```python
from build123d import *

# Parameters (mm, degrees)
F0_W     = 25.4
F0_H     = 6.604
F1_DEPTH = 3.175
F0_H_2   = 13.716
F0_H_3   = 2.54
F2_DEPTH = 19.05
F3_R     = 12.69999
F4_R     = 1.5875
F5_DEPTH = 25.4
F6_R     = 1.5875
F7_DEPTH = 2.54


# Not quite as in the source:
# - a fillet or chamfer is up to 0.001 mm smaller than in the source, because OpenCascade refuses the exact size


with BuildPart() as f1:
    # F0 (on Top) → F1 (new body)
    with BuildSketch(Plane.XY):
        Rectangle(F0_W, F0_H)
    extrude(amount=F1_DEPTH)



with BuildPart() as f1b:
    # F0 (on Top) → F1, piece 2 (new body)
    with BuildSketch(Plane.XY):
        with Locations((0, 12.7)):
            Rectangle(F0_W, F0_H_2)
    extrude(amount=F1_DEPTH)


with BuildPart() as f1_1:
    add(f1.part)

    add(f1b.part)  # F2 merges F1b
    # F0 (on Top) → F2 (join)
    with BuildSketch(Plane.XY):
        with Locations((0, -4.572)):
            Rectangle(F0_W, F0_H_3)
        with Locations((0, 4.572)):
            Rectangle(F0_W, F0_H_3)
    extrude(amount=F2_DEPTH)

    # F3 (radius 12.7 in the source; OpenCascade refuses exactly that, so slightly less here)
    f3_edges = [f1_1.edges().sort_by_distance(p)[0] for p in [
        (12.7, -4.572, 19.05),
        (12.7, 4.572, 19.05),
        (-12.7, -4.572, 19.05),
        (-12.7, 4.572, 19.05),
        (12.7, 19.558, 1.5875),
        (-12.7, 19.558, 1.5875),
    ]]
    fillet(f3_edges, radius=F3_R)

    # F4 (on face) → F5 (cut)
    with BuildSketch(Plane.XY.offset(3.175)):
        with Locations((0, 12.7)):
            Circle(F4_R)
    extrude(amount=-F5_DEPTH, mode=Mode.SUBTRACT)

    # F6 (on face) → F7 (cut, through all)
    with BuildSketch(Plane(origin=(0, 5.842, 0), x_dir=(-1, 0, 0), z_dir=(0, 1, 0))):
        with Locations((0, 10.033)):
            Circle(F6_R)
    extrude(amount=-F7_DEPTH, mode=Mode.SUBTRACT)


solid = f1_1.part
```
The listing builds one solid part. Answer for the finished solid, in the listing's coordinates (mm). A direction names the side the tool comes from. Coordinates: 2 decimals unless noted, no trailing zeros. Loops run counter-clockwise (first coordinate to the right, second up) from the corner with the lowest first, then second, coordinate; pieces in that order, holes last. Notation, with made-up numbers: (-3.5, -3) - (26.5, -3) arc R24 cw to (26.5, 29) - close; hole circle Ø5 at (-7.75, 0). An arc over 180 degrees is marked (long way). Write item = value, one per line.
1) Find the intervals of material crossed by line 1 along Y through (x, z) = (6, 10.5); line 2 along Y through (x, z) = (0, 1.3); line 3 along Z through (x, y) = (0, 4.55), in increasing order.
Responses:
line_1 = -5.84 to -3.3, 3.3 to 5.84
line_2 = -5.84 to 11.11, 14.29 to 19.56
line_3 = 0 to 8.45, 11.62 to 19.05
2) Section C-C (y = 12.7) is taken. Determine the outline of the cut face in (x, z) (1 decimal), plus the area to 3 significant figures.
Responses:
outline = (-11.3, 0) - (-1.6, 0) - (-1.6, 3.2) - (-11.3, 3.2) - close; (1.6, 0) - (11.3, 0) - (11.3, 3.2) - (1.6, 3.2) - close
area = 61.5 mm^2
3) Determine the mould class of faces 4 (the face through (-0.207, 14.274, 1.61)), 5 (the face through (0, 10, 3.175)), 6 (the face through (9.08, 15.74, 1.61)) for opening direction Y: pulls with the +Y half, pulls with the -Y half, needs draft (parallel to the pull), parting line crosses it, or undercut.
Responses:
face_4 = undercut
face_5 = needs draft
face_6 = pulls with the +Y half
4) Each of these flat-tipped pins is pushed along its axis until it touches: P1, Ø1, axis at x = -0.5, y = 12, coming from the +Z side; P2, Ø2.5, axis at x = 0, z = 10.033, coming from the +Y side; P3, Ø5, axis at x = 5, z = 9, coming from the +Y side; P4, Ø4, axis at x = 0, y = 12.7, coming from the +Z side (3 decimals). Where does it stop, or does it pass through?
Responses:
P1 = through
P2 = -3.3
P3 = 5.84
P4 = 3.175
5) Section D-D (z = 15.5) is taken. Determine the outline of the cut face in (x, y), plus the area to 3 significant figures.
Responses:
outline = (-8.81, -5.84) - (8.81, -5.84) - (8.81, -3.3) - (-8.81, -3.3) - close; (-8.81, 3.3) - (8.81, 3.3) - (8.81, 5.84) - (-8.81, 5.84) - close
area = 89.5 mm^2
6) Which of the six approach directions +Z, -Z, +X, -X, +Y, -Y give full straight-line access (tool end or side, diameter ignored) to faces 1 (the face through (0.207, 4.59, 11.607)), 2 (the face through (0, 5.842, 7)), 3 (the face through (0, -3.302, 9))?
Responses:
face_1 = +Y
face_2 = +Z, +X, -X, +Y
face_3 = +Z, +X, -X
7) Section B-B (x = 0.5) is taken. Determine the outline of the cut face in (y, z) (3 decimals).
Responses:
outline = (-5.842, 0) - (11.193, 0) - (11.193, 3.175) - (5.842, 3.175) - (5.842, 8.526) - (3.302, 8.526) - (3.302, 3.175) - (-3.302, 3.175) - (-3.302, 19.04) - (-5.842, 19.04) - close; (3.302, 11.54) - (5.842, 11.54) - (5.842, 19.04) - (3.302, 19.04) - close; (14.207, 0) - (19.548, 0) - (19.548, 3.175) - (14.207, 3.175) - close
